Build history of the part. All positions in model axes, mm. Give positions to 0.01 mm unless a question says otherwise; leave off trailing zeros. Order: outer loops, then holes, each group sorted by start corner. A loop starts at its lowest first (then second) coordinate and runs counter-clockwise, first axis right, second up. Notation, with made-up numbers: (-24, 5.5) - (29, 5.5) arc R19 cw to (29, 36.5) - close; hole circle Ø1 at (17.5, 11.5). An arc over 180 degrees is marked (long way). Write each question's results on one line, items separated by ' | '. Start each with the question number.
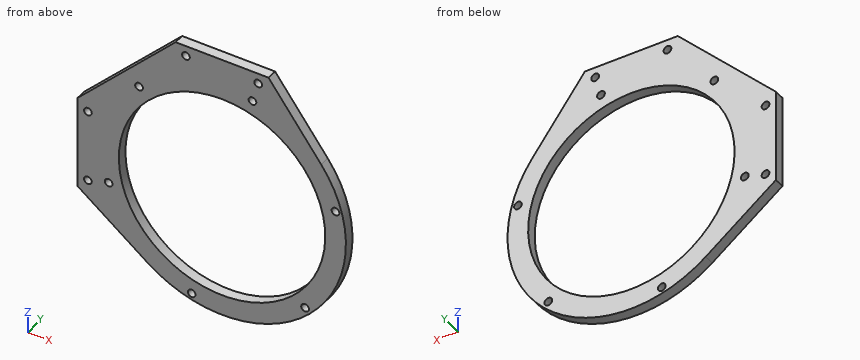
from build123d import *

# Parameters (mm, degrees)
SKETCH_1_R      = 40
SKETCH_1_R_2    = 1.5
EXTRUDE_1_DEPTH = 4


with BuildPart() as part:
    # 草图1 → 凸台-拉伸1 (new body)
    with BuildSketch(Plane(origin=(0, 0, 0), x_dir=(1, 0, 0), z_dir=(0, 1, 0))):
        with BuildLine():
            Line((-56, 18), (-56, -18))
            Line((-56, -18), (-18, -56))
            Line((-18, -56), (18, -56))
            Line((18, -56), (38.4, -28.8))
            ThreePointArc((38.4, -28.8), (33.941125497, 33.941125497), (-28.8, 38.4))
            Line((-28.8, 38.4), (-56, 18))
        make_face()
        with Locations(Location((0, 0, 0), (0, 0, 270))):
            Circle(SKETCH_1_R, mode=Mode.SUBTRACT)
        with Locations(Location((32.173358544, 32.173358544, 0), (0, 0, 270))):
            Circle(SKETCH_1_R_2, mode=Mode.SUBTRACT)
        with Locations(Location((43.949625096, -11.776266552, 0), (0, 0, 270))):
            Circle(SKETCH_1_R_2, mode=Mode.SUBTRACT)
        with Locations(Location((11.776266552, -43.949625096, 0), (0, 0, 270))):
            Circle(SKETCH_1_R_2, mode=Mode.SUBTRACT)
        with Locations(Location((-32.173358544, -32.173358544, 0), (0, 0, 270))):
            Circle(SKETCH_1_R_2, mode=Mode.SUBTRACT)
        with Locations(Location((-43.949625096, 11.776266552, 0), (0, 0, 270))):
            Circle(SKETCH_1_R_2, mode=Mode.SUBTRACT)
        with Locations(Location((-11.776266552, 43.949625096, 0), (0, 0, 270))):
            Circle(SKETCH_1_R_2, mode=Mode.SUBTRACT)
        with Locations(Location((-14, -52, 0), (0, 0, 270))):
            Circle(SKETCH_1_R_2, mode=Mode.SUBTRACT)
        with Locations(Location((14, -52, 0), (0, 0, 90))):
            Circle(SKETCH_1_R_2, mode=Mode.SUBTRACT)
        with Locations(Location((-52, -14, 0), (0, 0, 90))):
            Circle(SKETCH_1_R_2, mode=Mode.SUBTRACT)
        with Locations(Location((-52, 14, 0), (0, 0, 270))):
            Circle(SKETCH_1_R_2, mode=Mode.SUBTRACT)
    extrude(amount=EXTRUDE_1_DEPTH)


solid = part.part
Item 1: Flat gauge pins, fed straight in: pin 1 Ø2.5 at (x, z) = (-11.78, -43.95) entering from -Y; pin 2 Ø1 at (x, y) = (1.5, 2) entering from -Z; pin 3 Ø2 at (y, z) = (3.5, 25) entering from +X; pin 4 Ø4 at (x, z) = (-14, 52) entering from +Y. Where does each tip first touch, or does it go through?
Item 2: Probe line 1 along X through (y, z) = (2.6, 14.5); line 2 along Z through (x, y) = (-33.5, 1.45) (1 decimal); line 3 along Z through (x, y) = (-12, 0.3). List the from-to ranges inside material, lowest first. Write a range as from..to.
Item 3: Cut at C-C, the plane x = 0. List the corners of the cut face in (y, z).
Item 4: Cut at B-B, the plane z = 52. List the corners of the cut face in (x, y).
Item 5: Cut at D-D, the plane z = 1.5. List the corners of the cut face in (x, y).
Item 6: Cut at A-A, the plane x = -52. List the corners of the cut face in (y, z).
Values found:
1) pin 1: passes through | pin 2: stops at z = -47.99 | pin 3: stops at x = 41.57 | pin 4: stops at y = 4
2) line 1: x = -56..-53.41, -50.59..-37.28, 37.28..45.76 | line 2: z = -34.9..-21.9, 21.9..31.5, 32.9..40.5 | line 3: z = -46.48..-45.43, -42.47..-38.16, 38.16..56
3) outline: (0, -48) - (4, -48) - (4, -40) - (0, -40) - close; (0, 40) - (4, 40) - (4, 56) - (0, 56) - close
4) outline: (-22, 0) - (-15.5, 0) - (-15.5, 4) - (-22, 4) - close; (-12.5, 0) - (12.5, 0) - (12.5, 4) - (-12.5, 4) - close; (15.5, 0) - (21, 0) - (21, 4) - (15.5, 4) - close
5) outline: (-56, 0) - (-39.97, 0) - (-39.97, 4) - (-56, 4) - close; (39.97, 0) - (47.98, 0) - (47.98, 4) - (39.97, 4) - close
6) outline: (0, -21) - (4, -21) - (4, -15.5) - (0, -15.5) - close; (0, -12.5) - (4, -12.5) - (4, 12.5) - (0, 12.5) - close; (0, 15.5) - (4, 15.5) - (4, 22) - (0, 22) - close
